Part model, mm, in its own coordinate system. Face numbers are marked on the shaded views. Give positions to 0.01 mm unless a question says otherwise; leave off trailing zeros. Write each loop counter-clockwise with the first axis right and the second up, starting at its lowest first coordinate (ties: lowest second). Pieces come first, ordered by that corner, then holes.
from build123d import *

# Parameters (mm, degrees)
SKIZZE1_W                       = 9.5
SKIZZE1_H                       = 4
SKIZZE1_W_2                     = 2
SKIZZE1_H_2                     = 3
AUFSATZ_LINEAR_AUSTRAGEN4_DEPTH = 30
KREISMUSTER3_COUNT              = 2
SKIZZE3_W                       = 14
SKIZZE3_H                       = 3
SKIZZE3_W_2                     = 22.5
FASE1_SIZE                      = 1
FASE2_SIZE                      = 0.5


with BuildPart() as part:
    # Skizze1 → Rotation1 (revolve)
    with BuildSketch(Plane.XY, mode=Mode.PRIVATE) as rotation1_sk:
        with Locations((-22.75, -2)):
            Rectangle(SKIZZE1_W, SKIZZE1_H)
        with Locations((-23.5, -5.5)):
            Rectangle(SKIZZE1_W_2, SKIZZE1_H_2)
    revolve(rotation1_sk.sketch.rotate(Axis((0, -13.508693245, 0), (0, 1, 0)), 270), axis=Axis((0, -13.508693245, 0), (0, 1, 0)))

    # Skizze2 → Aufsatz-Linear austragen4 (add)
    with BuildSketch(Plane(origin=(0, 0, 0), x_dir=(0, 0, -1), z_dir=(1, 0, 0))):
        Polygon((-7.5, -7), (-7.5, -6), (7.5, -5), (7.5, -7), align=None)
    aufsatz_linear_austragen4 = extrude(amount=AUFSATZ_LINEAR_AUSTRAGEN4_DEPTH)

    # Kreismuster3: Aufsatz-Linear austragen4 ×2 about axis
    kreismuster3_axis = Axis((0, 0, 0), (0, 1, 0))
    for i in range(1, KREISMUSTER3_COUNT):
        add(aufsatz_linear_austragen4.rotate(kreismuster3_axis, i * 360 / KREISMUSTER3_COUNT))

    # Skizze3 → Schnitt-Rotation1 (revolve, cut)
    with BuildSketch(Plane.XY, mode=Mode.PRIVATE) as schnitt_rotation1_sk:
        with Locations((-33, -5.5)):
            Rectangle(SKIZZE3_W, SKIZZE3_H)
        with Locations((-11.25, -5.5)):
            Rectangle(SKIZZE3_W_2, SKIZZE3_H)
    revolve(schnitt_rotation1_sk.sketch.rotate(Axis((0, 1.410628136, 0), (0, -1, 0)), 90), axis=Axis((0, 1.410628136, 0), (0, -1, 0)), mode=Mode.SUBTRACT)

    # Fase1
    fase1_edges = [part.edges().sort_by_distance(p)[0] for p in [
        (0, -4, 22.5),
    ]]
    chamfer(fase1_edges, length=FASE1_SIZE)

    # Fase2
    fase2_edges = [part.edges().sort_by_distance(p)[0] for p in [
        (0, 0, 27.5),
        (0, -7, 22.5),
        (0, 0, 18),
        (0, -4, 18),
        (0, -4, 27.5),
    ]]
    chamfer(fase2_edges, length=FASE2_SIZE)


solid = part.part
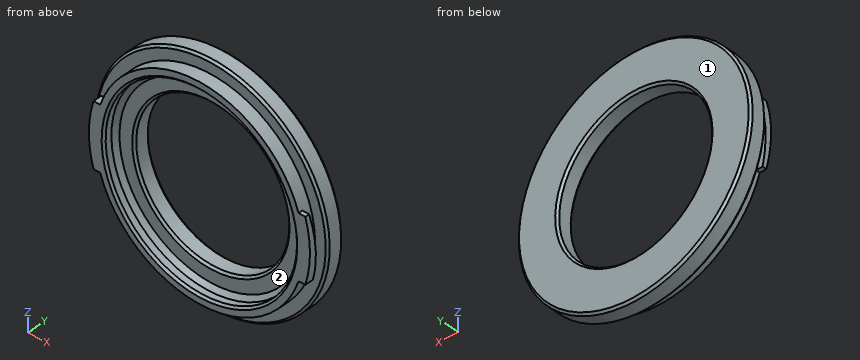
1) Flat gauge pins, fed straight in: P1, Ø4, axis at x = 21, y = -4, coming from the -Z side; P2, Ø5, axis at x = 9, z = -13, coming from the +Y side; P3, Ø2, axis at y = -5.5, z = -6, coming from the +X side. Where does each tip first touch, or does it go through?
Check result:
P1: stops at z = -19.82
P2: stops at y = -0.19
P3: stops at x = 25.51
2) Saw through at A-A (x = 0). Write the cut outline in (y, z), and give its area (4 significant figures).
Check result:
outline: (-7, -24.5) - (-4, -24.5) - (-4, -27) - (-3.5, -27.5) - (-0.5, -27.5) - (0, -27) - (0, -18.5) - (-0.5, -18) - (-3.5, -18) - (-4, -18.5) - (-4, -21.5) - (-5, -22.5) - (-6.5, -22.5) - (-7, -23) - close; (-7, 23) - (-6.5, 22.5) - (-5, 22.5) - (-4, 21.5) - (-4, 18.5) - (-3.5, 18) - (-0.5, 18) - (0, 18.5) - (0, 27) - (-0.5, 27.5) - (-3.5, 27.5) - (-4, 27) - (-4, 24.5) - (-7, 24.5) - close
area: 87.75 mm2
3) Drill centre lines: L1, parallel to X at y = -1.7, z = 0; L2, parallel to X at y = -5.45, z = 0; L3, parallel to Y at x = -4, z = 25. Where is each one in solid material? Low to high.
Check result:
L1: x = -27.5 to -18, 18 to 27.5
L2: x = -24.5 to -22.5, 22.5 to 24.5
L3: y = -4 to 0
4) Mould opens along Z. For the marked faces 1 and 2 say: +Z half, -Z half, draft (parallel to the pull), parting line (faces both ways), or undercut.
Check result:
face 1: draft
face 2: undercut
